Model file for the job. Use its own axes, mm. A direction names the side the tool comes from. Give positions to 0.01 mm unless a question says otherwise; leave off trailing zeros. Write each loop counter-clockwise with the first axis right and the second up, starting at its lowest first coordinate (ties: lowest second). Pieces come first, ordered by that corner, then holes. Notation, with made-up numbers: M -18,81.25 L 29,81.25 A37 cw 29,119.25 Z; hole C 53.5,-39 d10. An arc over 180 degrees is marked long. Answer as a JSON object with one key per item and string values. Group by question number.
```python
from build123d import *

# Parameters (mm, degrees)
SKETCH1_R           = 38.1
BOSS_EXTRUDE1_DEPTH = 12.7
SKETCH2_R           = 19.05
BOSS_EXTRUDE2_DEPTH = 25.4
SKETCH3_R           = 6.35
CUT_EXTRUDE1_DEPTH  = 66.991135768
SKETCH4_R           = 1.27
CUT_EXTRUDE2_DEPTH  = 6.35
SKETCH5_R           = 9.525
CUT_EXTRUDE3_DEPTH  = 1.5875


with BuildPart() as part:
    # Sketch1 → Boss-Extrude1 (new body)
    with BuildSketch(Plane(origin=(0, 0, 0), x_dir=(0, 0, -1), z_dir=(1, 0, 0))):
        Circle(SKETCH1_R)
    extrude(amount=BOSS_EXTRUDE1_DEPTH)

    # Sketch2 → Boss-Extrude2 (add)
    with BuildSketch(Plane(origin=(12.7, 0, 0), x_dir=(0, 0, -1), z_dir=(1, 0, 0))):
        Circle(SKETCH2_R)
    extrude(amount=BOSS_EXTRUDE2_DEPTH)

    # Sketch3 → Cut-Extrude1 (cut, through all)
    with BuildSketch(Plane(origin=(38.1, 0, 0), x_dir=(0, 0, -1), z_dir=(1, 0, 0))):
        Circle(SKETCH3_R)
    extrude(amount=-CUT_EXTRUDE1_DEPTH, mode=Mode.SUBTRACT)

    # Sketch4 → Cut-Extrude2 (cut)
    with BuildSketch(Plane(origin=(38.1, 0, 0), x_dir=(0, 0, -1), z_dir=(1, 0, 0))):
        with Locations((0, 13.583482333)):
            Circle(SKETCH4_R)
        with Locations((11.763640772, -6.791741166)):
            Circle(SKETCH4_R)
        with Locations((-11.763640772, -6.791741166)):
            Circle(SKETCH4_R)
    extrude(amount=-CUT_EXTRUDE2_DEPTH, mode=Mode.SUBTRACT)

    # Sketch5 → Cut-Extrude3 (cut)
    with BuildSketch(Plane(origin=(38.1, 0, 0), x_dir=(0, 0, -1), z_dir=(1, 0, 0))):
        Circle(SKETCH5_R)
        Polygon((-15.715448212, 11.225320151), (-11.225320151, 15.715448212), (2.24506403, 2.24506403), (-2.24506403, -2.24506403), align=None)
        Polygon((15.715448212, 11.225320151), (2.24506403, -2.24506403), (-2.24506403, 2.24506403), (11.225320151, 15.715448212), align=None)
    extrude(amount=-CUT_EXTRUDE3_DEPTH, mode=Mode.SUBTRACT)


solid = part.part
```
Q1. Wall check: L1, parallel to Y at x = 36, z = 0; L2, parallel to Z at x = 37.65, y = 0 (3 decimals); L3, parallel to X at y = -7, z = -28. Give the ranges that are in metal, low to high.
Q2. Drop flat-ended pins along their axis: P1, Ø3, axis at x = 8.5, y = 25.5, coming from the +Z side; P2, Ø1, axis at y = -9.5, z = -19.5, coming from the +X side; P3, Ø1, axis at x = 18.5, y = -10.5, coming from the -Z side. Give the stop position or say it passes through.
Q3. Slice it at C-C, the plane x = 23.5. Write the cut outline in (y, z), then the cut area to 3 significant figures.
Q4. 3-axis set-ups, long thin cutter, end or side, ignore diameter. For faces 4 (the flat face through (38.1, -10, 0)), 5 (the flat face through (31.75, 14, 0)): which of +Z, -Z, +X, -X, +Y, -Y reach the whole face in a straight line?
Q5. Slice it at D-D, the plane y = -24. Write the cut outline in (x, z), then the cut area to 3 significant figures.
Q6. Two-plate mould, pull along Z, no slides. Class faces 1 (the cylindrical face through (6.261, -23.183, 30.235)), 2 (the flat face through (12.7, 17.5, -7.9)), 3 (the flat face through (31.75, -7, -12)): +Z half, -Z half, draft (parallel to the pull), parting line (faces both ways), or undercut.
Solved:
{
 "1": {"L1": "y = -19.05 to -6.35, 6.35 to 12.31, 14.85 to 19.05", "L2": "z = -19.05 to -9.525, 9.525 to 19.05", "L3": "x = 0 to 12.7"},
 "2": {"P1": "stops at z = 29.59", "P2": "stops at x = 12.7", "P3": "stops at z = -16.21"},
 "3": {"outline": "C 0,0 d38.1; hole C 0,0 d12.7", "area": "1,010 mm²"},
 "4": {"face 4": "+Z, -Z, +X, +Y, -Y", "face 5": "+X"},
 "5": {"outline": "M 0,-29.59 L 12.7,-29.59 L 12.7,29.59 L 0,29.59 Z", "area": "752 mm²"},
 "6": {"face 1": "parting line", "face 2": "draft", "face 3": "undercut"}
}
